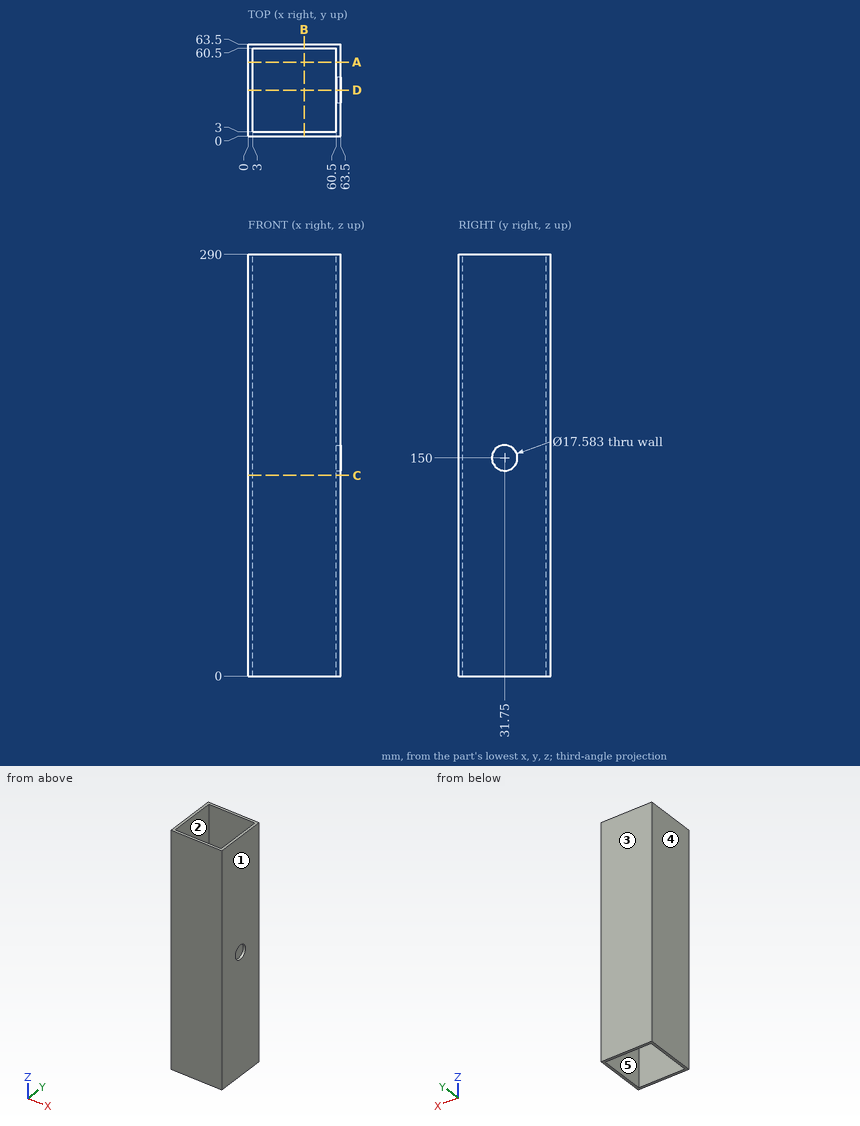
Part print with two shaded views. Sizes in mm from the minimum x, y, z corner. A direction names the side the tool comes from. Round coordinates to 2 decimals unless told otherwise and drop trailing zeros. Write each loop counter-clockwise with the first axis right and the second up, starting at its lowest first coordinate (ties: lowest second). Pieces come first, ordered by that corner, then holes. Notation, with made-up numbers: M 63.5,62.5 L 118.5,62.5 A28 cw 118.5,99.5 Z; hole C 13,4 d6. An arc over 180 degrees is marked long. Put each result on its own line as item: value. Start each with the question number.
1) Drill centre lines: probe 1 along X at (y, z) = (51, 168); probe 2 along Z at (x, y) = (62, 31). Where is each one in solid material? Low to high. Write a range as [from, to].
2) 3-axis set-ups, long thin cutter, end or side, ignore diameter. For the marked faces 4 and 5: which of +Z, -Z, +X, -X, +Y, -Y reach the whole face in a straight line?
3) Saw through at C-C, the plane z = 138. Write the cut outline in (x, y), and give its area (3 significant figures).
4) Pull direction X, two halves, no side cores. Call the marked faces 1, 2 and 3: pulls with the +X half, pulls with the -X half, needs draft (parallel to the pull), parting line crosses it, or undercut.
5) Saw through at A-A, the plane y = 51. Write the cut outline in (x, z).
6) Saw through at D-D, the plane y = 31.75. Write the cut outline in (x, z), and give its area (3 significant figures).
7) Pin check, flat tip, straight feed: pin 1 Ø12 at (y, z) = (41.5, 38.5) entering from -X. Stop position of the tip, or through.
Resolved:
1. probe 1: [0, 3], [60.5, 63.5]
1. probe 2: [0, 141.24], [158.76, 290]
2. face 4: +Z, -Z, -X, +Y, -Y
2. face 5: +Z, -Z
3. outline: M 0,0 L 63.5,0 L 63.5,63.5 L 0,63.5 Z; hole M 3,3 L 60.5,3 L 60.5,60.5 L 3,60.5 Z
3. area: 726 mm²
4. face 1: pulls with the +X half
4. face 2: undercut
4. face 3: needs draft
5. outline: M 0,0 L 3,0 L 3,290 L 0,290 Z; M 60.5,0 L 63.5,0 L 63.5,290 L 60.5,290 Z
6. outline: M 0,0 L 3,0 L 3,290 L 0,290 Z; M 60.5,0 L 63.5,0 L 63.5,141.21 L 60.5,141.21 Z; M 60.5,158.79 L 63.5,158.79 L 63.5,290 L 60.5,290 Z
6. area: 1,690 mm²
7. pin 1: x = 0
